Work out the finished part from the listing and answer in its coordinate system (mm). A direction names the side the tool comes from. Give positions to 0.01 mm unless a question says otherwise; leave off trailing zeros. Loops run counter-clockwise (first coordinate to the right, second up) from the corner with the lowest first, then second, coordinate; pieces in that order, holes last. Notation, with made-up numbers: M 22,-37.5 L 77,-37.5 A23 cw 77,-29.5 Z; hole C 6.25,82.5 d7. An arc over 180 degrees is marked long. Use a Markdown table: item, result.
```python
from build123d import *

# Parameters (mm, degrees)
EXTRUDE_1_DEPTH       = 378
CUT_EXTRUDE_1_DEPTH   = 379.956461879
HOLE_WIZARD_M31_D     = 3.4
HOLE_WIZARD_M31_DEPTH = 5
HOLE_WIZARD_M31_TIP   = 1.021463052


with BuildPart() as part:
    # Эскиз1 → Вытянуть-Тонкостенный1 (new body)
    with BuildSketch(Plane.XY):
        Polygon((20, 0), (0, 0), (0, 20), (2, 20), (2, 2), (20, 2), align=None)
    extrude(amount=EXTRUDE_1_DEPTH)

    # Эскиз2 → Вырез-Вытянуть1 (cut, through all)
    with BuildSketch(Plane(origin=(0, 2, 0), x_dir=(1, 0, 0), z_dir=(0, 1, 0))):
        with BuildLine():
            Line((7.5, -378), (7.5, -345.5))
            ThreePointArc((7.5, -345.5), (11.161165235, -336.661165235), (20, -333))
            Line((20, -333), (20, -378))
            Line((20, -378), (7.5, -378))
        make_face()
        with BuildLine():
            Line((20, 0), (7.5, 0))
            Line((7.5, 0), (7.5, -32.5))
            ThreePointArc((7.5, -32.5), (11.161165235, -41.338834765), (20, -45))
            Line((20, -45), (20, 0))
        make_face()
    extrude(amount=-CUT_EXTRUDE_1_DEPTH, mode=Mode.SUBTRACT)

    # Отверстие с зазором M31
    with Locations(Plane.XZ):
        with Locations((10, 50), (10, 84.75), (10, 119.5), (10, 154.25), (10, 189), (10, 223.75), (10, 258.5), (10, 293.25), (10, 328)):
            Hole(HOLE_WIZARD_M31_D / 2, depth=HOLE_WIZARD_M31_DEPTH)
            with Locations((0, 0, -(HOLE_WIZARD_M31_DEPTH + HOLE_WIZARD_M31_TIP / 2))):  # 118° drill point
                Cone(0, HOLE_WIZARD_M31_D / 2, HOLE_WIZARD_M31_TIP, mode=Mode.SUBTRACT)


solid = part.part
```
(1) A cutting plane is placed at B-B (y = 13). Write down the section's boundary in (x, z), and give its area (3 significant figures).
Entries:
| item | result |
|---|---|
| outline | M 0,0 L 2,0 L 2,378 L 0,378 Z |
| area | 756 mm² |
(2) A cutting plane is placed at A-A (z = 204). Write down the section's boundary in (x, y), and give its area (3 significant figures).
Entries:
| item | result |
|---|---|
| outline | M 0,0 L 20,0 L 20,2 L 2,2 L 2,20 L 0,20 Z |
| area | 76.0 mm² |
(3) Given P1, Ø6, axis at y = 16.5, z = 268.5, coming from the -X side; P2, Ø9, axis at y = 9.5, z = 199.5, coming from the +X side; P3, Ø2, axis at x = 10, z = 203.5, coming from the +Y side; P4, Ø1, axis at y = 1, z = 13.5, coming from the +X side, each flat-ended and moving along its own axis, determine where each tip first touches the part or whether it passes through.
Entries:
| item | result |
|---|---|
| P1 | stops at x = 0 |
| P2 | stops at x = 2 |
| P3 | stops at y = 2 |
| P4 | stops at x = 7.5 |
(4) Consider probe 1 along X at (y, z) = (0.55, 84.75); probe 2 along Y at (x, z) = (13.5, 188.5). Determine where each line is inside the solid, lowest interval first. Write a range as [from, to].
Entries:
| item | result |
|---|---|
| probe 1 | x = [0, 8.3], [11.7, 20] |
| probe 2 | y = [0, 2] |
(5) Which of the six approach directions +Z, -Z, +X, -X, +Y, -Y give full straight-line access (tool end or side, diameter ignored) to faces 1 (the flat face through (2, 11, 186)), 2 (the flat face through (10, 0, 186))?
Entries:
| item | result |
|---|---|
| face 1 | +Z, -Z, +X, +Y |
| face 2 | +Z, -Z, +X, -X, -Y |
(6) A cutting plane is placed at C-C (x = 16). Write down the section's boundary in (y, z), and give its area (3 significant figures).
Entries:
| item | result |
|---|---|
| outline | M 0,44.34 L 2,44.34 L 2,333.66 L 0,333.66 Z |
| area | 579 mm² |
